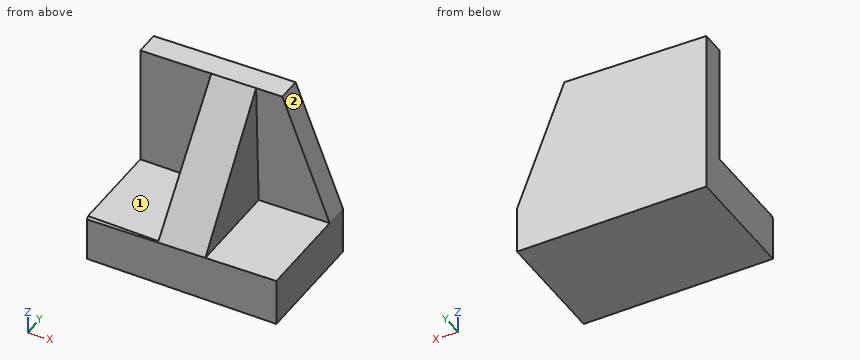
```python
from build123d import *

# Parameters (mm, degrees)
F1_DEPTH = 31.75
F3_DEPTH = 25.4
F5_DEPTH = 32.0061992138


with BuildPart() as f1:
    # F0 (on Front) → F1 (new body)
    with BuildSketch(Plane.XZ):
        Polygon((-19.3872701909, 48.5464597168), (-57.4788887117, 47.7473361589), (-57.4788887117, 3.2973361589), (-6.6788887117, 3.2973361589), (-6.6788887117, 15.9973361589), align=None)
    extrude(amount=F1_DEPTH)

    # F2 (on face) → F3 (cut)
    with BuildSketch(Plane.XZ.offset(31.75)):
        Polygon((-38.4288887117, 15.59777438), (-38.4288887117, 48.1469858553), (-57.4788887117, 47.7473361589), (-57.4788887117, 15.59777438), align=None)
        Polygon((-25.7246979722, 15.59777438), (-6.6788887117, 15.9973361589), (-19.3872701909, 48.5464597168), (-26.4128359261, 48.3990704667), align=None)
    extrude(amount=-F3_DEPTH, mode=Mode.SUBTRACT)

    # F4 (on face) → F5 (cut, through all)
    with BuildSketch(Plane(origin=(-25.3862995067, 0, -0.5325788394), x_dir=(0, 1, 0), z_dir=(0.9997800137, 0, 0.0209743716))):
        Polygon((-31.75, 16.1339024573), (-6.35, 48.9424159686), (-31.75, 48.9424159686), align=None)
    extrude(amount=-F5_DEPTH, mode=Mode.SUBTRACT)


solid = f1.part
```
Can you work these out from the model? Positions are in its coordinate system, mm. Face numbers are marked on the shaded views. A direction names the side the tool comes from. Give positions to 0.01 mm unless a question says otherwise; leave off trailing zeros. Order: outer loops, then holes, each group sorted by start corner. A loop starts at its lowest first (then second) coordinate and runs counter-clockwise, first axis right, second up. Notation, with made-up numbers: (6.25, 70) - (13.25, 70) arc R16 cw to (13.25, 95) - close; hole circle Ø8 at (69, -19). An arc over 180 degrees is marked (long way). Use a Markdown table: item, result. Add a question column.
Q1. If we section it at A-A on y = -5: Write out the boundary of the cut face in (x, z), plus the area to 3 significant figures.
Q2. If we section it at D-D on y = -23.5: Write out the boundary of the cut face in (x, z).
Q3. If we section it at C-C on x = -42: Write out the boundary of the cut face in (y, z).
Q4. On a 3-axis mill with a long thin cutter (end or side, diameter ignored), from which of +Z, -Z, +X, -X, +Y, -Y can I reach the whole of each face in a straight line? I mean the marked faces 1 and 2. Say none if no direction works.
Q5. If we section it at B-B on z = 32: Write out the boundary of the cut face in (x, y).
Q6. Please list where these lines run through material, in increasing order: line 1 along Z through (x, y) = (-53, -12); line 2 along Y through (x, z) = (-43, 38); line 3 along Z through (x, y) = (-27, -3).
Q7. I'm going to push flat-ended pins straight in: pin 1 (3 mm diameter, centred on y = -11, z = 32, fed in from -X); pin 2 (5.5 mm diameter, centred on x = -50.5, y = -20, fed in from +Z); pin 3 (2 mm diameter, centred on x = -37.5, z = 30.5, fed in from +Y). Where does each tip first touch, or does it pass through?
Answers follow:
| question | item | result |
|---|---|---|
| 1 | outline | (-57.48, 3.3) - (-6.68, 3.3) - (-6.68, 16) - (-19.39, 48.55) - (-57.48, 47.75) - close |
| 1 | area | 2,080 mm^2 |
| 2 | outline | (-57.48, 3.3) - (-6.68, 3.3) - (-6.68, 16) - (-25.72, 15.6) - (-25.95, 26.25) - (-38.43, 25.99) - (-38.43, 15.6) - (-57.48, 15.6) - close |
| 3 | outline | (-31.75, 3.3) - (0, 3.3) - (0, 48.07) - (-6.35, 48.07) - (-6.35, 15.6) - (-31.49, 15.6) - (-31.75, 15.26) - close |
| 4 | face 1 | +Z, -X, -Y |
| 4 | face 2 | +Z, +X, +Y, -Y |
| 5 | outline | (-57.48, -6.35) - (-38.43, -6.35) - (-38.43, -18.85) - (-26.07, -19.05) - (-26.07, -6.35) - (-12.93, -6.35) - (-12.93, 0) - (-57.48, 0) - close |
| 6 | line 1 | z = 3.3 to 15.6 |
| 6 | line 2 | y = -6.35 to 0 |
| 6 | line 3 | z = 3.3 to 48.39 |
| 7 | pin 1 | stops at x = -38.43 |
| 7 | pin 2 | stops at z = 15.6 |
| 7 | pin 3 | stops at y = 0 |
